Check sheet for the modelled part. Datum: model origin and axes. Units: mm. A direction names the side the tool comes from. Coordinates: 2 decimals unless noted, no trailing zeros. Order: outer loops, then holes, each group sorted by start corner. A loop starts at its lowest first (then second) coordinate and runs counter-clockwise, first axis right, second up.
from build123d import *

# Parameters (mm, degrees)
F0_W     = 59
F0_H     = 59
F1_DEPTH = 11.5
F2_R     = 5.74999
F4_DEPTH = 1
F6_DEPTH = 1


# Not quite as in the source:
# - a fillet or chamfer is up to 0.001 mm smaller than in the source, because OpenCascade refuses the exact size


with BuildPart() as f1:
    # F0 (on Top) → F1 (new body)
    with BuildSketch(Plane.XY):
        with Locations((29.5, -29.5)):
            Rectangle(F0_W, F0_H)
    extrude(amount=F1_DEPTH)

    # F2 (radius 5.75 in the source; OpenCascade refuses exactly that, so slightly less here)
    f2_edges = [f1.edges().sort_by_distance(p)[0] for p in [
        (29.5, -59, 11.5),
        (29.5, -59, 0),
        (29.5, 0, 11.5),
        (29.5, 0, 0),
    ]]
    fillet(f2_edges, radius=F2_R)

    # F3 (on face) → F4 (cut)
    with BuildSketch(Plane.YZ.offset(59)):
        with BuildLine():
            ThreePointArc((-5.75, 0.5999998897), (-0.5999998897, 5.75), (-5.75, 10.9000001103))
            Line((-5.75, 10.9000001103), (-53.25, 10.9000001103))
            ThreePointArc((-53.25, 10.9000001103), (-58.4000001103, 5.75), (-53.25, 0.5999998897))
            Line((-53.25, 0.5999998897), (-5.75, 0.5999998897))
        make_face()
    extrude(amount=-F4_DEPTH, mode=Mode.SUBTRACT)

    # F5 (on face) → F6 (cut)
    with BuildSketch(Plane(origin=(0, 0, 0), x_dir=(0, -1, 0), z_dir=(-1, 0, 0))):
        with BuildLine():
            Line((53.25, 10.9), (5.75, 10.9))
            ThreePointArc((5.75, 10.9), (0.6, 5.75), (5.75, 0.6))
            Line((5.75, 0.6), (53.25, 0.6))
            ThreePointArc((53.25, 0.6), (58.4, 5.75), (53.25, 10.9))
        make_face()
    extrude(amount=-F6_DEPTH, mode=Mode.SUBTRACT)


solid = f1.part
(1) Go/stop test with flat-tipped pins: P1, Ø3, axis at y = -38, z = 8, coming from the -X side; P2, Ø4, axis at y = -6, z = 9.5, coming from the +X side. Record where each tip stops, or that it passes through.
Filled in:
P1: stops at x = 1
P2: stops at x = 59
(2) Tool access check on faces 1 (the flat face through (29, -29, 11.5)), 2 (the cylindrical face through (58.51, -58.4, 5.86)), 3 (the flat face through (1, -29, 6)). Record the directions out of +Z, -Z, +X, -X, +Y, -Y that give a thin tool (end or side, any length) a straight path to the whole face; none if there is none.
Filled in:
face 1: +Z, +X, -X, +Y, -Y
face 2: +X
face 3: -X
(3) Thickness scan on probe 1 along X at (y, z) = (-36, 1.5); probe 2 along Y at (x, z) = (52, 6.25); probe 3 along Y at (x, z) = (33, 9.25). Record the ranges inside material, lowest first.
Filled in:
probe 1: x = 1 to 58
probe 2: y = -58.98 to -0.02
probe 3: y = -57.81 to -1.19
(4) Cross-section at C-C (z = 3.75). Enter the section's corners in (x, y), and give its area (3 significant figures).
Filled in:
outline: (0, -58.64) - (59, -58.64) - (59, -58) - (58, -58) - (58, -1) - (59, -1) - (59, -0.36) - (0, -0.36) - (0, -1) - (1, -1) - (1, -58) - (0, -58) - close
area: 3,320 mm2
(5) Cross-section at A-A (y = -45). Enter the section's corners in (x, z).
Filled in:
outline: (0, 0) - (59, 0) - (59, 0.6) - (58, 0.6) - (58, 10.9) - (59, 10.9) - (59, 11.5) - (0, 11.5) - (0, 10.9) - (1, 10.9) - (1, 0.6) - (0, 0.6) - close
(6) Release check for a two-part mould opening along Z. For faces 4 (the flat face through (29, -29, 0)), 5 (the flat face through (58, -30, 6)), 6 (the flat face through (59, -29.6, 11.3)), 7 (the cylindrical face through (0.49, -0.6, 5.86)) record: +Z half, -Z half, draft (parallel to the pull), parting line (faces both ways), or undercut.
Filled in:
face 4: -Z half
face 5: undercut
face 6: draft
face 7: undercut
